Input: dimensioned drawing with shaded views. Units: mm. Origin: part minimum x, y, z. A direction names the side the tool comes from. Give positions to 0.01 mm unless a question says otherwise; leave off trailing zeros. Loops run counter-clockwise (first coordinate to the right, second up) from the corner with the lowest first, then second, coordinate; pieces in that order, holes last. Notation, with made-up numbers: (-19.5, 76.5) -> (23.5, 76.5) arc R36 cw to (23.5, 113.5) -> close; hole circle Ø5 at (43, -30.5). An arc over 180 degrees is marked (long way). Answer as a JSON object with one key per item and string values.
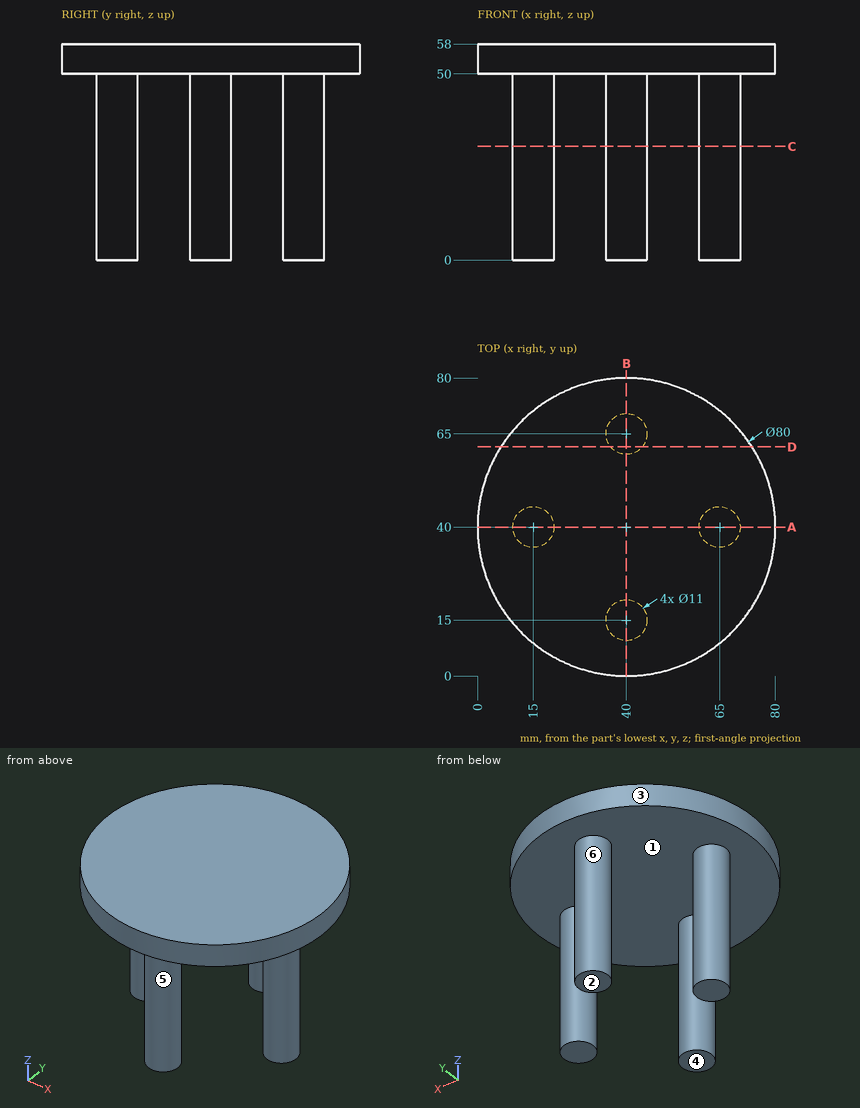
Q1. Ray query, line 1 along Z through (x, y) = (56, 53); line 2 along Y through (x, z) = (42.5, 48.5); line 3 along Y through (x, z) = (16.5, 48). Return the intervals inside material, ascending.
Evaluation:
{"line 1": "z = 50 to 58", "line 2": "y = 10.1 to 19.9, 60.1 to 69.9", "line 3": "y = 34.71 to 45.29"}
Q2. Section C-C, the plane z = 30.5. Return the cut outline in (x, y).
Evaluation:
{"outline": "circle Ø11 at (15, 40); circle Ø11 at (40, 15); circle Ø11 at (40, 65); circle Ø11 at (65, 40)"}
Q3. Section D-D, the plane y = 61.5. Return the cut outline in (x, z).
Evaluation:
{"outline": "(6.27, 50) -> (35.76, 50) -> (35.76, 0) -> (44.24, 0) -> (44.24, 50) -> (73.73, 50) -> (73.73, 58) -> (6.27, 58) -> close"}
Q4. Draft query along Y for the marked faces 3, 4, 5 and 6. Return one class per face: +Y half, -Y half, draft (parallel to the pull), parting line (faces both ways), or undercut.
Evaluation:
{"face 3": "parting line", "face 4": "draft", "face 5": "undercut", "face 6": "undercut"}
Q5. Access query for the marked faces 1 and 2. Directions: +Z, -Z, +X, -X, +Y, -Y. A direction counts if a zero-diameter tool reaches every point of the face in a straight line with its end or side. Return the directions, or none.
Evaluation:
{"face 1": "-Z", "face 2": "-Z, +X, -X, +Y, -Y"}
Q6. Section A-A, the plane y = 40. Return the cut outline in (x, z), then the cut area to 3 significant figures.
Evaluation:
{"outline": "(0, 50) -> (9.5, 50) -> (9.5, 0) -> (20.5, 0) -> (20.5, 50) -> (59.5, 50) -> (59.5, 0) -> (70.5, 0) -> (70.5, 50) -> (80, 50) -> (80, 58) -> (0, 58) -> close", "area": "1,740 mm2"}
Q7. Pin query (flat end, axial travel): pin 1 (1 mm diameter, centred on x = 10.5, z = 41, fed in from +Y); pin 2 (2 mm diameter, centred on x = 13, z = 51.5, fed in from -Y); pin 3 (6 mm diameter, centred on x = 41, z = 13, fed in from -Y). Return the tip coordinate at first contact, or that it passes through.
Evaluation:
{"pin 1": "stops at y = 43.77", "pin 2": "stops at y = 9.6", "pin 3": "stops at y = 9.5"}
